Here's how the part is built. I have some questions about the finished solid (model axes, mm). A direction names the side the tool comes from. Give positions to 0.01 mm unless a question says otherwise; leave off trailing zeros. Loops run counter-clockwise (first coordinate to the right, second up) from the corner with the lowest first, then second, coordinate; pieces in that order, holes last. Notation, with made-up numbers: M 45.5,58 L 100.5,58 A19 cw 100.5,73 Z; hole C 35.25,-39.75 d8. An arc over 180 degrees is marked long. Answer as CSV lines item,"result". Start each with the question number.
Item 1: If I drill on line 1 along Z through (x, y) = (-40, -32) (3 decimals); line 2 along Z through (x, y) = (-0.9, 5.5); line 3 along X through (y, z) = (-22, 14.5), over which ranges is the centre line in solid material (lowest first)? Write a range as from..to.
Item 2: I want a section at C-C on y = 5.5. List the corners of the cut face in (x, z) for me, plus the area to 3 significant figures.
Item 3: I want a section at B-B on x = -40. List the corners of the cut face in (y, z) for me (3 decimals), plus the area to 3 significant figures.
Item 4: I want a section at D-D on x = -6.5. List the corners of the cut face in (y, z) for me, plus the area to 3 significant figures.
Item 5: Will these pins go through, and if not, where does the flat tip stop? P1, Ø4, axis at x = -16, z = 10.5, coming from the +Y side; P2, Ø2, axis at y = -24.5, z = 6.5, coming from the -X side; P3, Ø3, axis at y = -2, z = 23.5, coming from the -X side.
Item 6: I want a section at A-A on y = -19. List the corners of the cut face in (x, z) for me, plus the area to 3 significant figures.
Item 7: If we mould it in two halves opening along Y, with no side actions, what happens to faces 6 (the flat face through (-9, 0, 0)), 7 (the flat face through (-83, -21, 0)), 8 (the flat face through (-91, -29, 0)), 9 (the flat face through (-81, -32, 36))? For each: released by +Y, released by -Y, zero draft, split by the parting line, or undercut.
Item 8: For faces 1 (the flat face through (-53, -33, 0)), 2 (the flat face through (-81, -32, -36)), 3 (the flat face through (-4, 6, 0)), 4 (the cylindrical face through (-12.435, -31.129, -6.655)), 5 (the flat face through (-9, -4, 0)), which set-ups out of +Z, -Z, +X, -X, +Y, -Y let a thin tool reach every point of the face, with its end or its side?
from build123d import *

# Parameters (mm, degrees)
EXTRUDE_BASE_DEPTH              = 32
SKETCH2_R                       = 2.2
SKETCH2_R_2                     = 2.2479
CUT_BOLT_HOLES_DEPTH            = 10
CUT_BOLT_HEAD_INSETS_DEPTH      = 40
CUT_BOLT_HEAD_INSETS_DEPTH_BACK = 4.2
SKETCH3_R                       = 4.215
SKETCH4_W                       = 40
SKETCH4_H                       = 3
CUT_TOP_CLEARANCE_SLOT_DEPTH    = 45
FILLET_CLEARANCE_SLOT_PT_1_R    = 3
FILLET_CLEARANCE_SLOT_PT_2_R    = 3
SKETCH5_R                       = 1.5
BOSS_EXTRUDE1_DEPTH             = 4
SKETCH6_R                       = 2.5
SKETCH7_R                       = 1.5
BOSS_EXTRUDE2_DEPTH             = 4
SKETCH9_R                       = 2.2479
BOSS_EXTRUDE3_DEPTH             = 4


with BuildPart() as part:
    # Sketch1 → Extrude-Base (new, symmetric)
    with BuildSketch(Plane.XY):
        Polygon((-14, 0), (0, 0), (0, -35), (-98, -35), (-98, -29), (-83, -29), (-83, -13), (-90, -13), (-90, -9), (-79, -9), (-79, -29), (-4, -29), (-4, -4), (-14, -4), align=None)
    extrude(amount=EXTRUDE_BASE_DEPTH, both=True)

    # Sketch2 → Cut-Bolt Holes (cut)
    with BuildSketch(Plane(origin=(0, -29, 0), x_dir=(1, 0, 0), z_dir=(0, 1, 0))):
        with Locations(Location((-15, -10, 0), (0, 0, 270))):
            Circle(SKETCH2_R)
        with Locations(Location((-15, 10, 0), (0, 0, 180))):
            Circle(SKETCH2_R)
        with Locations(Location((-40, 26.25, 0), (0, 0, 270))):
            Circle(SKETCH2_R_2)
        with Locations(Location((-40, -26.25, 0), (0, 0, 270))):
            Circle(SKETCH2_R_2)
    extrude(amount=-CUT_BOLT_HOLES_DEPTH, mode=Mode.SUBTRACT)

    # Sketch3 → Cut-Bolt Head Insets (cut, two sides: drawn at the far end of the back side and taken through both)
    with BuildSketch(Plane(origin=(0, -29, 0), x_dir=(1, 0, 0), z_dir=(0, 1, 0)).offset(-CUT_BOLT_HEAD_INSETS_DEPTH_BACK)):
        with Locations((-15, -10)):
            Circle(SKETCH3_R)
        with Locations((-40, -26.25)):
            Circle(SKETCH3_R)
        with Locations(Location((-15, 10, 0), (0, 0, 90))):
            Circle(SKETCH3_R)
        with Locations(Location((-40, 26.25, 0), (0, 0, 90))):
            Circle(SKETCH3_R)
    extrude(amount=CUT_BOLT_HEAD_INSETS_DEPTH + CUT_BOLT_HEAD_INSETS_DEPTH_BACK, mode=Mode.SUBTRACT)

    # Sketch4 → Cut-Top Clearance Slot (cut)
    with BuildSketch(Plane.ZY.offset(98)):
        with Locations((0, -33.5)):
            Rectangle(SKETCH4_W, SKETCH4_H)
    extrude(amount=-CUT_TOP_CLEARANCE_SLOT_DEPTH, mode=Mode.SUBTRACT)

    # Fillet-Clearance Slot Pt 1
    fillet_clearance_slot_pt_1_edges = [part.edges().sort_by_distance(p)[0] for p in [
        (-75.5, -32, 20),
        (-75.5, -32, -20),
    ]]
    fillet(fillet_clearance_slot_pt_1_edges, radius=FILLET_CLEARANCE_SLOT_PT_1_R - 0.0001)  # a hair under: the kernel refuses the full size

    # Fillet-Clearance Slot Pt 2
    # the kernel refuses this fillet: 3 mm, written as the material it takes off along each edge
    with BuildSketch(Plane(origin=(-103.490486718, -35, 20), x_dir=(0, 0, 1), z_dir=(1, 0, 0))) as fillet_clearance_slot_pt_2_piece_1:
        with BuildLine():
            CenterArc((2.196194687, -3), FILLET_CLEARANCE_SLOT_PT_2_R, 90, 60.000551337)
            Line((-0.401895958, -1.500025), (-0.661705022, -1.3500275))
            ThreePointArc((-0.661705022, -1.3500275), (-0.3, -0.0001), (-0.3, 0))
            Line((-0.3, 0), (0, 0.3))
            Line((0, 0.3), (2.196194687, 0.3))
            Line((2.196194687, 0.3), (2.196194687, 0))
        make_face()
    extrude(amount=50.490486718, mode=Mode.SUBTRACT)
    with BuildSketch(Plane(origin=(-103.490486718, -35, -20), x_dir=(0, 0.9659313848535173, 0.25879829936644894), z_dir=(1, 0, 0))) as fillet_clearance_slot_pt_2_piece_2:
        with BuildLine():
            CenterArc((2.329422704, -2.897768274), FILLET_CLEARANCE_SLOT_PT_2_R, 105.000679234, 60.000551337)
            Line((-0.56837145, -2.121373376), (-0.858150866, -2.043733886))
            Line((-0.858150866, -2.043733886), (-0.289779415, 0.07763949))
            Line((-0.289779415, 0.07763949), (0.07763949, 0.289779415))
            ThreePointArc((0.07763949, 0.289779415), (0.077736083, 0.289753536), (1.475282068, 0.289776827))
            Line((1.475282068, 0.289776827), (1.552931216, 0))
        make_face()
    extrude(amount=50.490486718, mode=Mode.SUBTRACT)

    # Sketch5 → Boss-Extrude1 (add)
    with BuildSketch(Plane.XY.offset(32)):
        with Locations(Location((-81, -32, 0), (0, 0, 180))):
            Circle(SKETCH5_R)
    extrude(amount=BOSS_EXTRUDE1_DEPTH)

    # Sketch6 → section 1 of loft2
    with BuildSketch(Plane.XY.offset(36), mode=Mode.PRIVATE) as loft2_s1:
        with Locations((-81, -32)):
            Circle(SKETCH6_R)
    # loft up to a face of the part (loft2)
    loft([Face(Wire([part.edges().sort_by_distance((-79.973179341, -33.093452941, 32))[0]])), loft2_s1.sketch])

    # Sketch7 → Boss-Extrude2 (add)
    with BuildSketch(Plane(origin=(0, 0, -32), x_dir=(-1, 0, 0), z_dir=(0, 0, -1))):
        with Locations((81, -32)):
            Circle(SKETCH7_R)
    extrude(amount=BOSS_EXTRUDE2_DEPTH)

    # Loft4: read off the stored shape, not the designer's step
    # Loft4: loft between two sections, ruled curve by curve
    loft4_from = [
        Edge.make_bspline([(-82.101258326, -29.755622559, -36), (-86.590013209, -31.95813921, -36), (-84.387496557, -36.446894093, -36), (-79.898741674, -34.244377441, -36), (-75.409986791, -32.04186079, -36), (-77.612503443, -27.553105907, -36), (-82.101258326, -29.755622559, -36)], [0, 0, 0, 0, 0.5, 0.5, 0.5, 1, 1, 1, 1], 3, [1, 0.333333333, 0.333333333, 1, 0.333333333, 0.333333333, 1]),
    ]
    loft4_to = [
        Edge.make_bspline([(-81.328134577, -30.536330741, -32), (-84.255473095, -31.192599896, -32), (-83.59920394, -34.119938413, -32), (-80.671865423, -33.463669259, -32), (-77.744526905, -32.807400104, -32), (-78.40079606, -29.880061587, -32), (-81.328134577, -30.536330741, -32)], [0, 0, 0, 0, 0.5, 0.5, 0.5, 1, 1, 1, 1], 3, [1, 0.333333333, 0.333333333, 1, 0.333333333, 0.333333333, 1]),
    ]
    loft4 = Solid(Shell([*[Face.make_surface_from_curves(loft4_from[k], loft4_to[k]) for k in range(1)], Face(Wire(loft4_from)), Face(Wire(loft4_to))]))
    add(loft4)

    # Sketch9 → Boss-Extrude3 (add)
    with BuildSketch(Plane(origin=(0, 0, 0), x_dir=(0, 0, -1), z_dir=(1, 0, 0))):
        with BuildLine():
            Line((32, 0), (-32, 0))
            Line((-32, 0), (-32, 7.5))
            ThreePointArc((-32, 7.5), (-30.535533906, 11.035533906), (-27, 12.5))
            Line((-27, 12.5), (27, 12.5))
            ThreePointArc((27, 12.5), (30.535533906, 11.035533906), (32, 7.5))
            Line((32, 7.5), (32, 0))
        make_face()
        with Locations(Location((-18, 5.5, 0), (0, 0, 90))):
            Circle(SKETCH9_R, mode=Mode.SUBTRACT)
        with Locations(Location((18, 5.5, 0), (0, 0, 90))):
            Circle(SKETCH9_R, mode=Mode.SUBTRACT)
    extrude(amount=-BOSS_EXTRUDE3_DEPTH)


solid = part.part
Result:
1,line 1,"-32..-30.465, -22.035..22.035, 30.465..32"
1,line 2,"-32..-20.25, -15.75..15.75, 20.25..32"
1,line 3,"-83..-79, -4..0"
2,outline,"M -4,-32 L 0,-32 L 0,-20.25 L -4,-20.25 Z; M -4,-15.75 L 0,-15.75 L 0,15.75 L -4,15.75 Z; M -4,20.25 L 0,20.25 L 0,32 L -4,32 Z"
2,area,"220 mm^2"
3,outline,"M -35,-32 L -29,-32 L -29,-30.465 L -33.2,-30.465 L -33.2,-28.498 L -35,-28.498 Z; M -35,-24.002 L -33.2,-24.002 L -33.2,-22.035 L -29,-22.035 L -29,22.035 L -33.2,22.035 L -33.2,24.002 L -35,24.002 Z; M -35,28.498 L -33.2,28.498 L -33.2,30.465 L -29,30.465 L -29,32 L -35,32 Z"
3,area,"297 mm^2"
4,outline,"M -35,-32 L -29,-32 L -29,32 L -35,32 Z; M -4,-32 L 0,-32 L 0,32 L -4,32 Z"
4,area,"640 mm^2"
5,P1,"y = -33.2"
5,P2,"x = -83"
5,P3,"x = -14"
6,outline,"M -83,-32 L -79,-32 L -79,32 L -83,32 Z; M -4,-32 L 0,-32 L 0,32 L -4,32 Z"
6,area,"512 mm^2"
7,face 6,"released by +Y"
7,face 7,"undercut"
7,face 8,"undercut"
7,face 9,"zero draft"
8,face 1,"-X, -Y"
8,face 2,"-Z, +X, -X, +Y, -Y"
8,face 3,"+Z, -Z, -X, +Y"
8,face 4,"+Y"
8,face 5,"+Z, -Z, -X"
